Check sheet for the drawn part. Datum: minimum x, y, z corner. Units: mm. Give positions to 0.01 mm unless a question says otherwise; leave off trailing zeros. Order: outer loops, then holes, each group sorted by start corner. A loop starts at its lowest first (then second) coordinate and runs counter-clockwise, first axis right, second up.
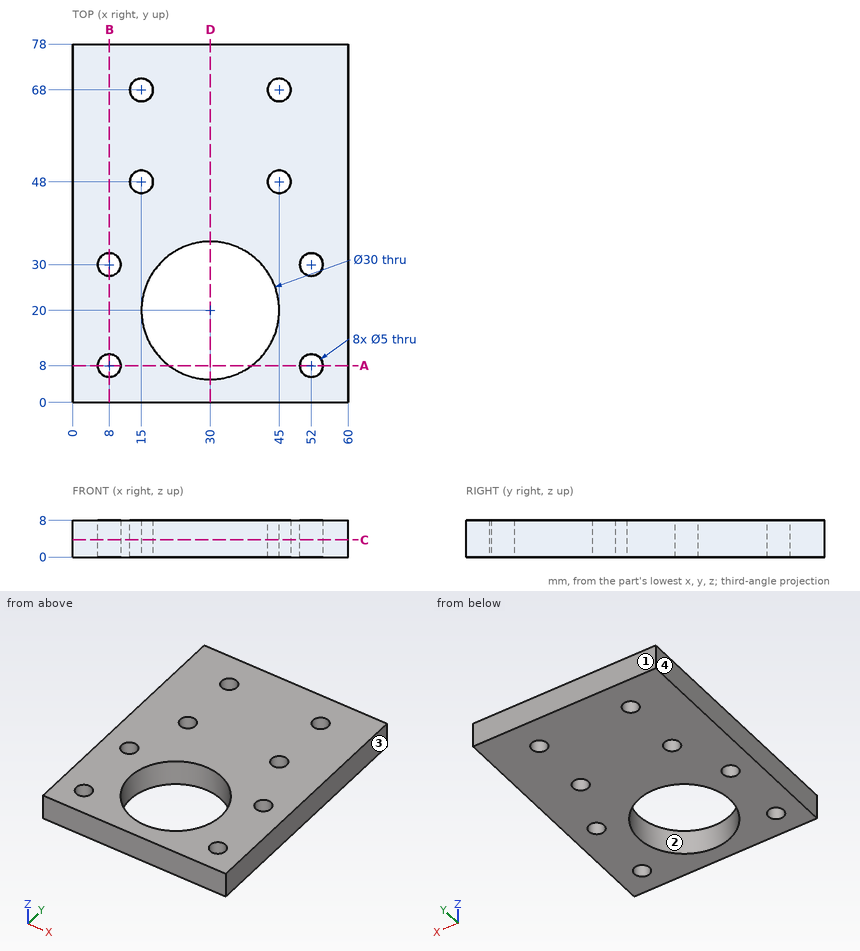
(1) Section check C-C, the plane z = 3.75. Give the number of separate pieces and of enclosed holes in the cut face, then the cut area to 3 significant figures.
Solved:
separate pieces: 1
enclosed holes: 9
area: 3,820 mm2
(2) Release check for a two-part mould opening along X. For the marked faces 1, 2, 3 and 4 record: pulls with the +X half, pulls with the -X half, needs draft (parallel to the pull), parting line crosses it, or undercut.
Solved:
face 1: needs draft
face 2: undercut
face 3: pulls with the +X half
face 4: pulls with the -X half
(3) Go/stop test with a flat-tipped pin: pin 1 (4.5 mm diameter, centred on x = 45, y = 48, fed in from -Z). Record where the tip stops, or that it passes through.
Solved:
pin 1: passes through
(4) Section check B-B, the plane x = 8. Enter the section's corners in (y, z).
Solved:
outline: (0, 0) - (5.5, 0) - (5.5, 8) - (0, 8) - close; (10.5, 0) - (27.5, 0) - (27.5, 8) - (10.5, 8) - close; (32.5, 0) - (78, 0) - (78, 8) - (32.5, 8) - close
(5) Section check D-D, the plane x = 30. Enter the section's corners in (y, z), then the cut area to 3 significant figures.
Solved:
outline: (0, 0) - (5, 0) - (5, 8) - (0, 8) - close; (35, 0) - (78, 0) - (78, 8) - (35, 8) - close
area: 384 mm2
(6) Scan lines: line 1 (X direction, y = 48, z = 5.75); line 2 (Y direction, x = 8, z = 3); line 3 (Y direction, x = 13.5, z = 2.25). Record each from-to range of solid material in increasing order.
Solved:
line 1: x = 0 to 12.5, 17.5 to 42.5, 47.5 to 60
line 2: y = 0 to 5.5, 10.5 to 27.5, 32.5 to 78
line 3: y = 0 to 46, 50 to 66, 70 to 78
(7) Section check A-A, the plane y = 8. Enter the section's corners in (x, z), then the cut area to 3 significant figures.
Solved:
outline: (0, 0) - (5.5, 0) - (5.5, 8) - (0, 8) - close; (10.5, 0) - (21, 0) - (21, 8) - (10.5, 8) - close; (39, 0) - (49.5, 0) - (49.5, 8) - (39, 8) - close; (54.5, 0) - (60, 0) - (60, 8) - (54.5, 8) - close
area: 256 mm2
